The model under review builds one solid part; all positions refer to its coordinate system, in mm. Round coordinates to 2 decimals unless told otherwise and drop trailing zeros. Order: outer loops, then holes, each group sorted by start corner. A loop starts at its lowest first (then second) coordinate and runs counter-clockwise, first axis right, second up. Notation, with made-up numbers: M 56.5,18 L 85.5,18 A17 cw 85.5,33 Z; hole C 61.5,-39 d10. An arc over 180 degrees is marked long. Answer as a JSON object with one key per item and string values. Group by question number.
1. Add section B-B on y = -7.75. State the section outline as (x, z) points, and give its area (3 significant figures).
2. To check wall thickness, follow probe 1 along Z at (x, y) = (336, -10.5); probe 2 along Z at (x, y) = (-341, -1.25); probe 3 along X at (y, z) = (-6.75, 1). State the ranges of each line that lie inside material, in increasing order. Write a range as [from, to].
3. Clearance check with flat-ended pins moving along their axes: P1, Ø2, axis at y = -4.5, z = -5, coming from the -X side; P2, Ø2, axis at y = -10.5, z = -28, coming from the +X side. State where each tip first meets the part, or that it passes through.
```python
from build123d import *

# Parameters (mm, degrees)
F0_W     = 1500
F0_H     = 75
F1_DEPTH = 12
F2_SIZE  = 11.99999


# Not quite as in the source:
# - a fillet or chamfer is up to 0.001 mm smaller than in the source, because OpenCascade refuses the exact size


with BuildPart() as f1:
    # F0 (on Front) → F1 (new body)
    with BuildSketch(Plane.XZ):
        Rectangle(F0_W, F0_H)
    extrude(amount=F1_DEPTH)

    # F2 (size 12 in the source; OpenCascade refuses exactly that, so slightly less here)
    f2_edges = [f1.edges().sort_by_distance(p)[0] for p in [
        (0, 0, 37.5),
        (750, 0, 0),
        (-750, 0, 0),
    ]]
    chamfer(f2_edges, length=F2_SIZE)


solid = f1.part
```
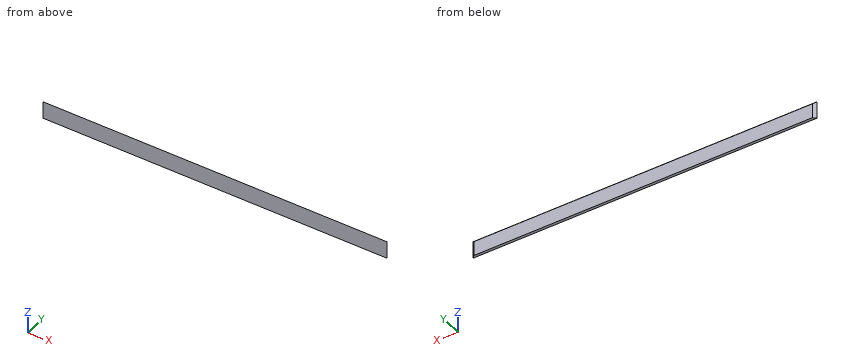
Recorded:
{
 "1": {"outline": "M -745.75,-37.5 L 745.75,-37.5 L 745.75,33.25 L -745.75,33.25 Z", "area": "106,000 mm²"},
 "2": {"probe 1": "z = [-37.5, 36]", "probe 2": "z = [-37.5, 26.75]", "probe 3": "x = [-744.75, 744.75]"},
 "3": {"P1": "stops at x = -743.5", "P2": "stops at x = 749.5"}
}
